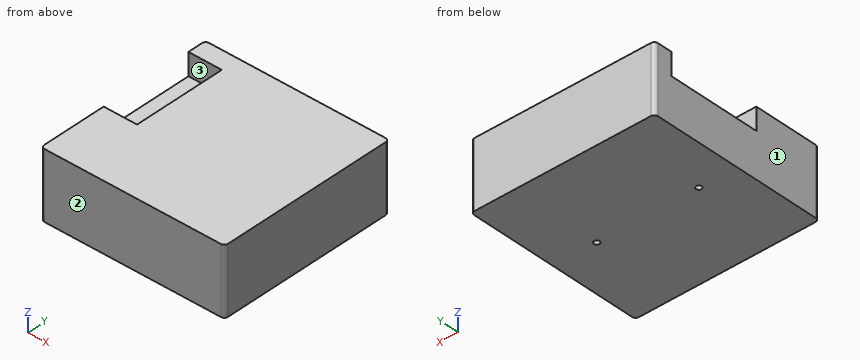
```python
from build123d import *

# Parameters (mm, degrees)
F0_W     = 99
F0_H     = 97
F1_DEPTH = 36
F2_R     = 1.5
F3_DEPTH = 3
F4_W     = 18
F4_H     = 50
F5_DEPTH = 12
F6_R     = 2


with BuildPart() as f1:
    # F0 (on Top) → F1 (new body)
    with BuildSketch(Plane.XY):
        Rectangle(F0_W, F0_H)
    extrude(amount=F1_DEPTH)

    # F2 (on face) → F3 (cut)
    with BuildSketch(Plane(origin=(0, 0, 0), x_dir=(1, 0, 0), z_dir=(0, 0, -1))):
        with Locations((-29, 0)):
            Circle(F2_R)
        with Locations((26, 0)):
            Circle(F2_R)
    extrude(amount=-F3_DEPTH, mode=Mode.SUBTRACT)

    # F4 (on face) → F5 (cut)
    with BuildSketch(Plane.XY.offset(36)):
        with Locations((-40.5, 13.5)):
            Rectangle(F4_W, F4_H)
    extrude(amount=-F5_DEPTH, mode=Mode.SUBTRACT)

    # F6
    f6_edges = [f1.edges().sort_by_distance(p)[0] for p in [
        (-49.5, -48.5, 18),
        (49.5, -48.5, 18),
        (49.5, 48.5, 18),
        (-49.5, 48.5, 18),
    ]]
    fillet(f6_edges, radius=F6_R)


solid = f1.part
```
CAD build for the part. Positions are in the model's coordinates, mm. Face numbers are marked on the shaded views. Round coordinates to 2 decimals unless told otherwise and drop trailing zeros. Write each loop counter-clockwise with the first axis right and the second up, starting at its lowest first coordinate (ties: lowest second). Pieces come first, ordered by that corner, then holes. Notation, with made-up numbers: (7.25, 82.5) - (34.25, 82.5) arc R27 ccw to (34.25, 100.5) - close; hole circle Ø2 at (83, -5). An arc over 180 degrees is marked (long way). Return JSON: item names as keys, results as strings. Group by question number.
Item 1: Flat gauge pins, fed straight in: pin 1 Ø9.5 at (y, z) = (18, 31.5) entering from -X; pin 2 Ø2.5 at (x, y) = (-29, 0) entering from -Z; pin 3 Ø5.5 at (x, y) = (-44.5, 7.5) entering from +Z. Where does each tip first touch, or does it go through?
Item 2: Band-saw the part on A-A on z = 30. List the corners of the cut face in (x, y), plus the area to 3 significant figures.
Item 3: Mould opens along Y. For the marked faces 1, 2 and 3 say: +Y half, -Y half, draft (parallel to the pull), parting line (faces both ways), or undercut.
Item 4: Probe probe 1 along X at (y, z) = (0, 2); probe 2 along Y at (x, z) = (-36, 30); probe 3 along Y at (x, z) = (26, 1.4). List the from-to ranges inside material, lowest first.
Item 5: Band-saw the part on B-B on x = -38.5. List the corners of the cut face in (y, z).
Resolved:
{
 "1": {"pin 1": "stops at x = -31.5", "pin 2": "stops at z = 3", "pin 3": "stops at z = 24"},
 "2": {"outline": "(-49.5, -46.5) arc R2 ccw to (-47.5, -48.5) - (47.5, -48.5) arc R2 ccw to (49.5, -46.5) - (49.5, 46.5) arc R2 ccw to (47.5, 48.5) - (-47.5, 48.5) arc R2 ccw to (-49.5, 46.5) - (-49.5, 38.5) - (-31.5, 38.5) - (-31.5, -11.5) - (-49.5, -11.5) - close", "area": "8,700 mm²"},
 "3": {"face 1": "draft", "face 2": "-Y half", "face 3": "undercut"},
 "4": {"probe 1": "x = -49.5 to -30.5, -27.5 to 24.5, 27.5 to 49.5", "probe 2": "y = -48.5 to -11.5, 38.5 to 48.5", "probe 3": "y = -48.5 to -1.5, 1.5 to 48.5"},
 "5": {"outline": "(-48.5, 0) - (48.5, 0) - (48.5, 36) - (38.5, 36) - (38.5, 24) - (-11.5, 24) - (-11.5, 36) - (-48.5, 36) - close"}
}
